Autodesk Inventor part; units mm, degrees
ref_plane "Work Plane2" through (0, 0, 0) normal (0, 0, 1) x (1, 0, 0)
ref_plane "YZ Plane" through (0, 0, 0) normal (1, 0, 0) x (0, 1, 0)
ref_plane "XZ Plane" through (0, 0, 0) normal (0, 1, 0) x (-1, 0, 0)
ref_plane "Work Plane1" through (0, 0, 0) normal (0, 0, 1) x (1, 0, 0)
ref_plane "Work Plane2" through (0, 0, 0) normal (0, 0, 1) x (1, 0, 0)
ref_plane "Work Plane3" through (18.3844, -18.3844, 0) normal (0.7071, 0.7071, 0) x (-0.7071, 0.7071, 0)
sketch "Sketch2" plane through (18.3844, -18.3844, 0) normal (0.7071, 0.7071, 0) x (-0.7071, 0.7071, 0)
  line L0 (2.9994, 0) -> (12.9994, 17.3205)
  line L1 (-4.0006, 0) -> (15.9994, 0) construction
  line L2 (48.9994, 0) -> (38.9994, 17.3205)
  line L3 (56.0448, 0) -> (76.0448, 0) construction
  line L4 (38.9994, 17.3205) -> (12.9994, 17.3205)
  line L5 (7.6182, 0) -> (15.3088, 13.3205)
  line L6 (15.3088, 13.3205) -> (36.69, 13.3205)
  line L7 (36.69, 13.3205) -> (44.3806, 0)
  line L8 (-17.6765, -6) -> (-19.9184, -71)
  line L9 (53.3865, -6) -> (55.409, -71)
  line L10 (20.5601, 2) -> (20.5601, 10)
  line L11 (33.5601, 2) -> (33.5601, 10)
  line L12 (48, 0) -> (-12, 0)
  line L13 (44.3806, 0) -> (48.9994, 0)
  line L14 (2.9994, 0) -> (7.6182, 0)
  line L15 (-4.0006, -9.8008) -> (-4.0006, -30.1937)
  line L16 (55.9994, -9.8008) -> (55.9994, -30.1937)
  point P0 (25.9994, 0)
  dimension "d1" = 20
  dimension "d2" = 60
  dimension "d3" = 120
  dimension "d5" = 4
  dimension "d6" = 4
  dimension "d7" = 4
  dimension "d24" = 7
  dimension "d25" = 7
extrude "Extrusion1" add sketch "Sketch2" along normal mid plane 20 contours L0 L4 L2 L13 L12 L7 L6 L5
sketch "Sketch3" plane through (16.2635, -2.1213, 17.3205) normal (0, 0, 1) x (0.7071, 0.7071, 0)
  circle A0 centre (-9.3718, 30.7817) radius 1.4
  circle A1 centre (-10.6281, -5.1964) radius 1.4
  line L0 (-20, -5.3812) -> (0, -5.3812)
  point P0 (-9.968, 30.7817)
  point P1 (-10, -5.3812)
hole "Hole1" at (-12.5509, 12.5962, 17.3205) at (12.9975, -12.9975, 17.3205) direction (0, 0, -1) diameter 2.8 end through all counterbore diameter 6.5 counterbore depth 12
sketch "Sketch4" plane through (16.2635, -2.1213, 17.3205) normal (0, 0, 1) x (0.7071, 0.7071, 0)
  circle A0 centre (-10.0015, 21.2913) radius 1.9
  line L0 (0, 26) -> (0, 0)
  line L1 (-20, 0) -> (-20, 26)
  circle A1 centre (-10.0015, 4.2912) radius 1.9
  circle A2 centre (-10.0015, 12.7912) radius 3
  circle A3 centre (-10.0015, 21.2913) radius 1.4
  circle A4 centre (-10.0015, 4.2912) radius 1.9
  circle A5 centre (-10.0015, 4.2912) radius 1.4
  line L2 (-20, 26) -> (0, 26)
  line L3 (-20, 0) -> (0, 0)
  point P0 (-10, 13)
  dimension "d17" = 2.8
  dimension "d18" = 2.8
extrude "Extrusion2" cut sketch "Sketch4" against normal blind 20 contours A2 | A3 | A5
ref_plane "Arbeitsebene4" through (18.3844, -18.3844, 0) normal (0.7071, 0.7071, 0) x (0, 0, 1)
properties part number "Anglerfish_Lightplate_Tislinkbridge"
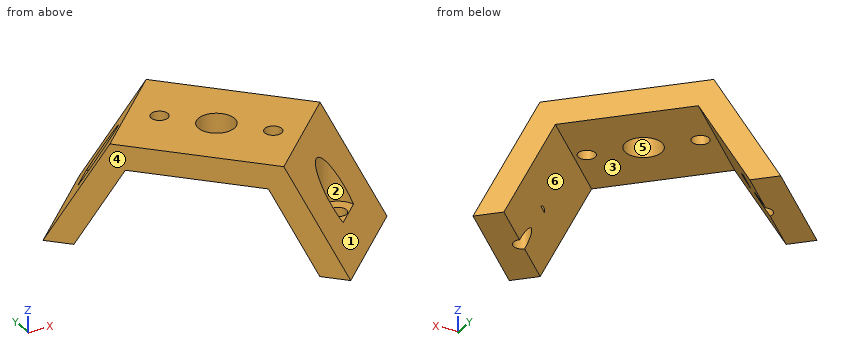
Build history of the part. All positions in model axes, mm. Face numbers are marked on the shaded views. A direction names the side the tool comes from. Round coordinates to 2 decimals unless told otherwise and drop trailing zeros. Loops run counter-clockwise (first coordinate to the right, second up) from the corner with the lowest first, then second, coordinate; pieces in that order, holes last. Notation, with made-up numbers: (5, -27.5) -> (43, -27.5) arc R23 cw to (43, -4.5) -> close; hole circle Ø8 at (-6.5, 55). An arc over 180 degrees is marked (long way). Use CSV: the item, a comma, the result in double quotes. Start each with the question number.
Q1. Which spindle directions (+Z, -Z, +X, -X, +Y, -Y) get a long thin tool onto all of the face, cutting with end or side? Do the marked faces 1, 2 and 3. Say none if no direction does.
Q2. Saw through at C-C on x = 17. Give the cut face in (y, z), and give its area (3 significant figures).
Q3. Saw through at D-D on y = -19.5. Give the cut face in (x, z), and give its area (3 significant figures).
Q4. Drill centre lines: L1, parallel to Z at x = 4, y = 7; L2, parallel to Y at x = 5, z = 14; L3, parallel to Y at x = -2.5, z = 16. Where is each one in solid material? Low to high.
Q5. Mould opens along Y. For the marked faces 4, 5 and 6 say: +Y half, -Y half, draft (parallel to the pull), parting line (faces both ways), or undercut.
Q6. Saw through at A-A on z = 8.25. Give the cut face in (x, y), and give its area (3 significant figures).
Q7. Saw through at B-B on z = 3.5. Give the cut face in (x, y).
Q8. Flat gauge pins, fed straight in: pin 1 Ø6 at (x, y) = (13, -13) entering from +Z; pin 2 Ø10 at (x, y) = (6, -1.5) entering from -Z; pin 3 Ø7.5 at (x, y) = (-12.55, 12.6) entering from +Z. Where does each tip first touch, or does it go through?
Solutions:
1,face 1,"+Z, +X, -Y"
1,face 2,"+Z"
1,face 3,"-Z"
2,outline,"(-15.53, 0) -> (-9, 0) -> (-2.86, 7.52) -> (-2.86, 15.52) -> close"
2,area,"75.2 mm^2"
3,outline,"(5.36, 1.39) -> (6.5, 0) -> (13.03, 0) -> (5.36, 9.39) -> close"
3,area,"35.2 mm^2"
4,L1,"z = 13.32 to 17.32"
4,L2,"y = -16.1 to -6.95, -5.37 to 9.14"
4,L3,"y = -11.64 to -1.56, 1.26 to 16.64"
5,face 4,"-Y half"
5,face 5,"undercut"
5,face 6,"+Y half"
6,outline,"(-19.97, 5.82) -> (-16.7, 2.56) -> (-2.56, 16.7) -> (-5.82, 19.97) -> (-10.6, 15.19) arc R3.25 cw (long way) to (-15.15, 10.64) -> close; (2.56, -16.7) -> (5.82, -19.97) -> (10.6, -15.19) arc R3.25 cw to (15.19, -10.6) -> (19.97, -5.82) -> (16.7, -2.56) -> close"
6,area,"150 mm^2"
7,outline,"(-21.91, 7.76) -> (-18.64, 4.5) -> (-4.5, 18.64) -> (-7.76, 21.91) -> close; (4.5, -18.64) -> (7.76, -21.91) -> (21.91, -7.76) -> (18.64, -4.5) -> close; hole circle Ø2.8 at (-12.55, 12.6); hole circle Ø2.8 at (13, -13)"
8,pin 1,"stops at z = 5.32"
8,pin 2,"stops at z = 13.32"
8,pin 3,"stops at z = 15.53"
